For this review, take the finished solid that the model builds, in its own axes (mm). A direction names the side the tool comes from. Coordinates: 2 decimals unless noted, no trailing zeros. Loops run counter-clockwise (first coordinate to the right, second up) from the corner with the lowest first, then second, coordinate; pieces in that order, holes last. Notation, with made-up numbers: (4, -8.5) - (33, -8.5) arc R23 cw to (33, 4.5) - close; hole circle Ø3 at (35.25, 30.25). An arc over 180 degrees is marked (long way). Use one line per item in the form item = value. Start each with the question number.
1. For pin 1 Ø3 at (x, y) = (-80, 17.5) entering from -Z; pin 2 Ø2 at (y, z) = (18, -69) entering from -X; pin 3 Ø0.8 at (y, z) = (17.5, -89.5) entering from +X, all flat-tipped, find the tip position at first contact; note any pin that passes through.
2. Add section A-A on z = -62. Give the boundary of the cut face in (x, y) (3 decimals), and give its area (3 significant figures).
3. Draft analysis for pull direction X (two halves, no side actions). For faces 3 (the face through (-88, 8, 0)), 4 (the face through (-176.89, 18.1, -51.51)), 5 (the face through (-60.57, 17.8, -68.63)), 6 (the face through (-60.57, 17.8, -30.53)), state which applies: +X half, -X half, draft (parallel to the pull), parting line (faces both ways), or undercut.
4. Add section D-D on x = -63.5. Count the separate pieces of the cut face and the enclosed holes in it, and give its area (3 significant figures).
5. Machinability: for faces 1 (the face through (-88, 8, -2.54)), 2 (the face through (-88.5, 0, -99.5)), which of the approach directions +Z, -Z, +X, -X, +Y, -Y give a long, thin tool a straight path to every point of the face, cutting with its end or side? Answer none if there is none.
6. Add section B-B on x = -132. Give the boundary of the cut face in (y, z) (3 decimals).
7. Add section C-C on y = 4. Give the boundary of the cut face in (x, z), and give its area (3 significant figures).
8. To check wall thickness, follow probe 1 along Z at (x, y) = (-156.5, 7.75); probe 2 along X at (y, z) = (4, -78.5); probe 3 along Z at (x, y) = (-63.5, 18.2) (3 decimals). State the ranges of each line that lie inside material, in increasing order.
Autodesk Inventor part; units mm, degrees
ref_plane "YZ Plane" through (0, 0, 0) normal (1, 0, 0) x (0, 1, 0)
ref_plane "XZ Plane" through (0, 0, 0) normal (0, 1, 0) x (-1, 0, 0)
ref_plane "XY Plane" through (0, 0, 0) normal (0, 0, 1) x (1, 0, 0)
sketch "Sketch1" plane through (0, 0, 0) normal (0, 1, 0) x (-1, 0, 0)
  line L0 (0, 0) -> (177.8, 0)
  line L1 (177.8, 0) -> (177.8, -101.6)
  line L2 (177.8, -101.6) -> (0, -101.6)
  line L3 (0, -101.6) -> (0, 0)
  point P0 (177.8, -50.8)
  point P1 (88.9, 0)
  point P2 (0, -50.8)
  dimension "d0" = 177.8
  dimension "d1" = 101.6
extrude "Extrusion1" add sketch "Sketch1" along normal blind 19.05
fillet "Fillet1" radius 3.175 4 edges at (-88.9, 19.05, 0) (-177.8, 19.05, -50.8) (-88.9, 19.05, -101.6) (0, 19.05, -50.8)
sketch "Sketch2" plane through (0, 19.05, 0) normal (0, 1, 0) x (1, 0, 0)
  line L0 (-170.815, 6.985) -> (-113.665, 6.985)
  line L1 (-113.665, 6.985) -> (-113.665, 94.615)
  line L2 (-113.665, 94.615) -> (-170.815, 94.615)
  line L3 (-170.815, 94.615) -> (-170.815, 6.985)
  line L4 (-177.8, 0) -> (0, 0)
  line L5 (-177.8, 101.6) -> (-177.8, 0)
  line L6 (-82.55, 9.525) -> (-76.2, 9.525)
  line L7 (-76.2, 9.525) -> (-76.2, 15.875)
  line L8 (-76.2, 15.875) -> (-82.55, 15.875)
  line L9 (-82.55, 15.875) -> (-82.55, 9.525)
  line L10 (0, 0) -> (0, 101.6)
  line L11 (-82.55, 28.575) -> (-76.2, 28.575)
  line L12 (-76.2, 28.575) -> (-76.2, 34.925)
  line L13 (-76.2, 34.925) -> (-82.55, 34.925)
  line L14 (-82.55, 34.925) -> (-82.55, 28.575)
  line L15 (-82.55, 47.625) -> (-76.2, 47.625)
  line L16 (-76.2, 47.625) -> (-76.2, 53.975)
  line L17 (-76.2, 53.975) -> (-82.55, 53.975)
  line L18 (-82.55, 53.975) -> (-82.55, 47.625)
  line L19 (-82.55, 66.675) -> (-76.2, 66.675)
  line L20 (-76.2, 66.675) -> (-76.2, 73.025)
  line L21 (-76.2, 73.025) -> (-82.55, 73.025)
  line L22 (-82.55, 73.025) -> (-82.55, 66.675)
  line L23 (-82.55, 85.725) -> (-76.2, 85.725)
  line L24 (-76.2, 85.725) -> (-76.2, 92.075)
  line L25 (-76.2, 92.075) -> (-82.55, 92.075)
  line L26 (-82.55, 92.075) -> (-82.55, 85.725)
  circle A0 centre (-63.5, 12.7) radius 3.175
  circle A1 centre (-63.5, 31.75) radius 3.175
  circle A2 centre (-63.5, 50.8) radius 3.175
  circle A3 centre (-63.5, 69.85) radius 3.175
  circle A4 centre (-63.5, 88.9) radius 3.175
  line L27 (0, 101.6) -> (-177.8, 101.6)
  point P0 (-79.375, 15.875)
  point P1 (-79.375, 28.575)
  point P2 (-79.375, 34.925)
  point P3 (-79.375, 47.625)
  dimension "d47" = 87.63
  dimension "d48" = 57.15
  dimension "d49" = 6.985
  dimension "d50" = 6.985
  dimension "d51" = 6.35
  dimension "d52" = 6.35
  dimension "d53" = 9.525
  dimension "d54" = 76.2
  dimension "d55" = 6.35
  dimension "d56" = 6.35
  dimension "d57" = 6.35
  dimension "d58" = 6.35
  dimension "d59" = 6.35
  dimension "d60" = 6.35
  dimension "d61" = 6.35
  dimension "d62" = 6.35
  dimension "d63" = 12.7
  dimension "d64" = 12.7
  dimension "d65" = 12.7
  dimension "d66" = 12.7
  dimension "d67" = 76.2
  dimension "d68" = 6.35
  dimension "d69" = 6.35
  dimension "d70" = 6.35
  dimension "d71" = 6.35
  dimension "d72" = 6.35
  dimension "d73" = 63.5
  dimension "d74" = 63.5
  dimension "d75" = 63.5
  dimension "d76" = 63.5
  dimension "d77" = 63.5
  dimension "d78" = 12.7
  dimension "d79" = 19.05
  dimension "d80" = 19.05
  dimension "d81" = 19.05
  dimension "d82" = 19.05
shell "Shell2" thickness 2.54 removed faces 1 at (-59.2667, 0, -33.8667)
extrude "Extrusion2" cut sketch "Sketch2" against normal blind 19.05 contours L3 L2 L1 L0 | L9 L8 L7 L6 | L14 L13 L12 L11 | L18 L17 L16 L15 | L22 L21 L20 L19 | L26 L25 L24 L23 | A0 | A1 | A2 | A3 | A4
properties part number "CaseTop" material "PC/ABS Plastic"
Conclusion:
q1.pin_1 = -101.6
q1.pin_2 = -177.59
q1.pin_3 = -0.25
q2.outline = (-177.8, 0) - (-175.26, 0) - (-175.26, 15.875) arc R0.635 cw to (-174.625, 16.51) - (-170.815, 16.51) - (-170.815, 19.05) - (-174.625, 19.05) arc R3.175 ccw to (-177.8, 15.875) - close; (-113.665, 16.51) - (-3.175, 16.51) arc R0.635 cw to (-2.54, 15.875) - (-2.54, 0) - (0, 0) - (0, 15.875) arc R3.175 ccw to (-3.175, 19.05) - (-113.665, 19.05) - close
q2.area = 386 mm^2
q3.face_3 = draft
q3.face_4 = -X half
q3.face_5 = undercut
q3.face_6 = undercut
q4.separate_pieces = 6
q4.enclosed_holes = 0
q4.area = 257 mm^2
q5.face_1 = -Y
q5.face_2 = +Z, -Z, +X, -X, -Y
q6.outline = (0, -101.6) - (15.875, -101.6) arc R3.175 ccw to (19.05, -98.425) - (19.05, -94.615) - (16.51, -94.615) - (16.51, -98.425) arc R0.635 cw to (15.875, -99.06) - (0, -99.06) - close; (0, -2.54) - (15.875, -2.54) arc R0.635 cw to (16.51, -3.175) - (16.51, -6.985) - (19.05, -6.985) - (19.05, -3.175) arc R3.175 ccw to (15.875, 0) - (0, 0) - close
q7.outline = (-177.8, -101.6) - (0, -101.6) - (0, 0) - (-177.8, 0) - close; hole (-175.26, -99.06) - (-2.54, -99.06) - (-2.54, -2.54) - (-175.26, -2.54) - close
q7.area = 1,390 mm^2
q8.probe_1 = -101.6 to -99.06, -2.54 to 0
q8.probe_2 = -177.8 to -175.26, -2.54 to 0
q8.probe_3 = -100.587 to -92.075, -85.725 to -73.025, -66.675 to -53.975, -47.625 to -34.925, -28.575 to -15.875, -9.525 to -1.013
